The model under review builds one solid part; all positions refer to its coordinate system, in mm. Face numbers are marked on the shaded views. Round coordinates to 2 decimals unless told otherwise and drop trailing zeros. Write each loop counter-clockwise with the first axis right and the second up, starting at its lowest first coordinate (ties: lowest second). Pieces come first, ordered by that corner, then holes. Notation, with made-up numbers: (24.25, 66) - (57.25, 66) arc R18 cw to (57.25, 88) - close; hole circle Ø1 at (-23, 60.5). An arc over 180 degrees is marked (long way). Write each question's results on one line, items separated by ' | '.
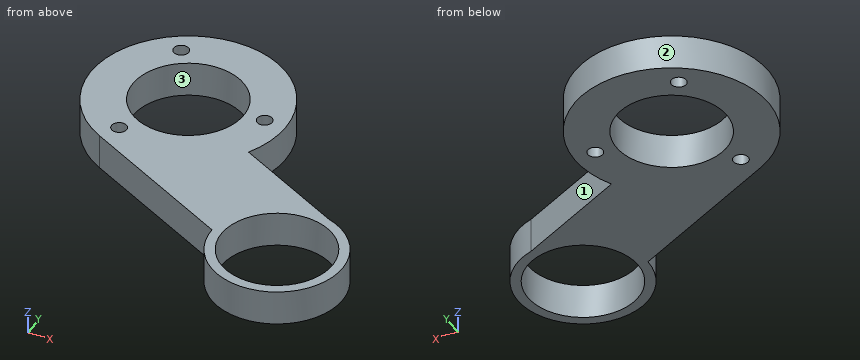
```python
from build123d import *

# Parameters (mm, degrees)
SKETCH1_R           = 1.5
SKETCH1_R_2         = 11
BOSS_EXTRUDE1_DEPTH = 7


with BuildPart() as part:
    # Sketch1 → Boss-Extrude1 (new body)
    with BuildSketch(Plane.XY):
        with BuildLine():
            Line((24.749447939, -15.649541482), (2.734486559, -4.010388703))
            ThreePointArc((2.734486559, -4.010388703), (-19.612688755, 23.883391477), (-23.148073161, -11.682888541))
            Line((-23.148073161, -11.682888541), (7.752714707, -28.019914292))
            ThreePointArc((7.752714707, -28.019914292), (28.40263196, -38.530802267), (24.749447939, -15.649541482))
        make_face()
        with Locations(Location((0.862954929, 5.91648973, 0), (0, 0, 180))):
            Circle(SKETCH1_R, mode=Mode.SUBTRACT)
        with Locations(Location((-21.15738061, -7.87136082, 0), (0, 0, 180))):
            Circle(SKETCH1_R, mode=Mode.SUBTRACT)
        with Locations(Location((-14.127422454, 5.37928778, 0), (0, 0, 180))):
            Circle(SKETCH1_R_2, mode=Mode.SUBTRACT)
        with Locations(Location((-22.08784168, 18.092734431, 0), (0, 0, 180))):
            Circle(SKETCH1_R, mode=Mode.SUBTRACT)
        with Locations(Location((20.752714707, -28.019914292, 0), (0, 0, 180))):
            Circle(SKETCH1_R_2, mode=Mode.SUBTRACT)
    extrude(amount=BOSS_EXTRUDE1_DEPTH)


solid = part.part
```
Q1. The part is to be moulded in two halves that separate along X. For the marked faces 1, 2 and 3, say which applies: released by +X, released by -X, zero draft, split by the parting line, or undercut.
Evaluation:
face 1: released by +X | face 2: split by the parting line | face 3: undercut
Q2. We need section D-D (y = -12.5). State the section outline as (x, z) points.
Evaluation:
outline: (-21.6, 0) - (18.79, 0) - (18.79, 7) - (-21.6, 7) - close
Q3. For probe 1 along Y at (x, z) = (-23, 1.5); probe 2 along X at (y, z) = (-28.5, 4.5); probe 3 along Y at (x, z) = (23.5, 6.75), list the stretches that pass through material, from the lowest coordinate up.
Evaluation:
probe 1: y = -11.76 to -1.12, 11.88 to 16.9, 19.28 to 22.52 | probe 2: x = 7.76 to 9.76, 31.74 to 33.74 | probe 3: y = -40.73 to -38.67, -17.37 to -14.99
Q4. We need section C-C (z = 1). State the section outline as (x, y) points, plus the area to 3 significant figures.
Evaluation:
outline: (-23.15, -11.68) - (7.75, -28.02) arc R13 ccw (long way) to (24.75, -15.65) - (2.73, -4.01) arc R19.3 ccw (long way) to start; hole circle Ø22 at (-14.13, 5.38); hole circle Ø3 at (-22.09, 18.09); hole circle Ø3 at (-21.16, -7.87); hole circle Ø3 at (0.86, 5.92); hole circle Ø22 at (20.75, -28.02) | area: 1,300 mm^2
Q5. Insertion check: P1, Ø3.5, axis at x = -22.09, y = 18.09, coming from the -Z side; P2, Ø4, axis at y = -5.5, z = 5.5, coming from the +X side; P3, Ø3, axis at y = -4.5, z = 1, coming from the +X side; P4, Ø2.5, axis at x = -21.16, y = -7.87, coming from the -Z side. Each pin has a flat end and moves straight along its axis. Give the tip position at first contact, or say it passes through.
Evaluation:
P1: stops at z = 0 | P2: stops at x = 9.33 | P3: stops at x = 6.5 | P4: passes through
Q6. We need section A-A (x = 22). State the section outline as (y, z) points, plus the area to 3 significant figures.
Evaluation:
outline: (-40.96, 0) - (-38.95, 0) - (-38.95, 7) - (-40.96, 7) - close; (-17.09, 0) - (-14.2, 0) - (-14.2, 7) - (-17.09, 7) - close | area: 34.3 mm^2
Q7. We need section B-B (y = -27). State the section outline as (x, z) points, plus the area to 3 significant figures.
Evaluation:
outline: (5.82, 0) - (9.8, 0) - (9.8, 7) - (5.82, 7) - close; (31.71, 0) - (33.71, 0) - (33.71, 7) - (31.71, 7) - close | area: 41.9 mm^2
